```python
from build123d import *

# Parameters (mm, degrees)
F0_W     = 45
F0_H     = 6
F1_DEPTH = 8
F2_W     = 10
F2_H     = 1.35
F3_DEPTH = 6.001
F4_R     = 1.5
F5_DEPTH = 8.001
F6_R     = 2


with BuildPart() as f1:
    # F0 (on Top) → F1 (new body)
    with BuildSketch(Plane.XY):
        Rectangle(F0_W, F0_H)
    extrude(amount=F1_DEPTH)

    # F2 (on face) → F3 (cut, through all)
    with BuildSketch(Plane.XZ.offset(3)):
        with BuildLine():
            Line((-19.25, 0), (-6.75, 0))
            ThreePointArc((-6.75, 0), (-13, 6.25), (-19.25, 0))
        make_face()
        with Locations((12, 0.675)):
            Rectangle(F2_W, F2_H)
    extrude(amount=-F3_DEPTH, mode=Mode.SUBTRACT)

    # F4 (on face) → F5 (cut, through all)
    with BuildSketch(Plane.XY.offset(8)):
        Circle(F4_R)
    extrude(amount=-F5_DEPTH, mode=Mode.SUBTRACT)

    # F6
    f6_edges = [f1.edges().sort_by_distance(p)[0] for p in [
        (-22.5, -3, 4),
        (-22.5, 3, 4),
        (22.5, -3, 4),
        (22.5, 3, 4),
    ]]
    fillet(f6_edges, radius=F6_R)


solid = f1.part
```
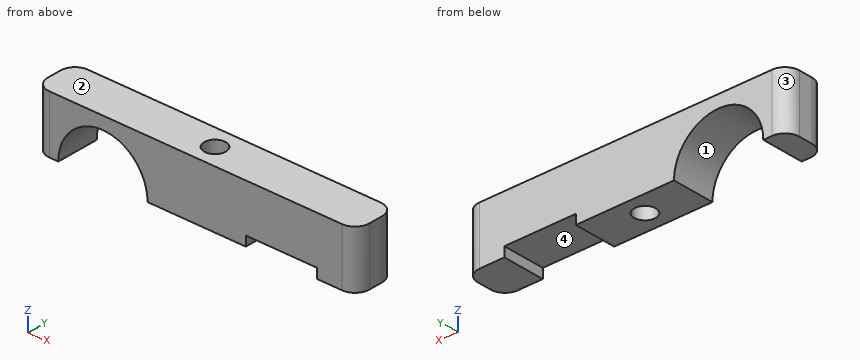
Model file for the job. Use its own axes, mm. Face numbers are marked on the shaded views. Coordinates: 2 decimals unless noted, no trailing zeros. Loops run counter-clockwise (first coordinate to the right, second up) from the corner with the lowest first, then second, coordinate; pieces in that order, holes last. Notation, with made-up numbers: (28.5, 5.25) -> (37.5, 5.25) arc R19 cw to (37.5, 33.25) -> close; hole circle Ø3 at (7.5, -2). An arc over 180 degrees is marked (long way). Answer as a JSON object with one key per item and string values.
Q1. Cut at D-D (y = -2). List the corners of the cut face in (x, z).
Report:
{"outline": "(-22.23, 0) -> (-19.25, 0) arc R6.25 cw to (-6.75, 0) -> (7, 0) -> (7, 1.35) -> (17, 1.35) -> (17, 0) -> (22.23, 0) -> (22.23, 8) -> (-22.23, 8) -> close"}
Q2. Cut at C-C (y = 0). List the corners of the cut face in (x, z).
Report:
{"outline": "(-22.5, 0) -> (-19.25, 0) arc R6.25 cw to (-6.75, 0) -> (-1.5, 0) -> (-1.5, 8) -> (-22.5, 8) -> close; (1.5, 0) -> (7, 0) -> (7, 1.35) -> (17, 1.35) -> (17, 0) -> (22.5, 0) -> (22.5, 8) -> (1.5, 8) -> close"}
Q3. Cut at B-B (x = 0). List the corners of the cut face in (y, z).
Report:
{"outline": "(-3, 0) -> (-1.5, 0) -> (-1.5, 8) -> (-3, 8) -> close; (1.5, 0) -> (3, 0) -> (3, 8) -> (1.5, 8) -> close"}
Q4. Cut at A-A (z = 5). List the corners of the cut face in (x, y).
Report:
{"outline": "(-22.5, -1) arc R2 ccw to (-20.5, -3) -> (-16.75, -3) -> (-16.75, 3) -> (-20.5, 3) arc R2 ccw to (-22.5, 1) -> close; (-9.25, -3) -> (20.5, -3) arc R2 ccw to (22.5, -1) -> (22.5, 1) arc R2 ccw to (20.5, 3) -> (-9.25, 3) -> close; hole circle Ø3 at (0, 0)"}
Q5. Probe probe 1 along Y at (x, z) = (0, 3.25); probe 2 along X at (y, z) = (0.5, 2); probe 3 along Z at (x, y) = (10.5, 2). List the from-to ranges inside material, lowest first.
Report:
{"probe 1": "y = -3 to -1.5, 1.5 to 3", "probe 2": "x = -22.5 to -18.92, -7.08 to -1.41, 1.41 to 22.5", "probe 3": "z = 1.35 to 8"}
Q6. Pull direction X, two halves, no side cores. Call the marked faces 1, 2, 3 and 4: released by +X, released by -X, zero draft, split by the parting line, or undercut.
Report:
{"face 1": "undercut", "face 2": "zero draft", "face 3": "released by -X", "face 4": "undercut"}
